Geometry check sheet. Reference: the model listing, model coordinates, mm. A direction names the side the tool comes from. Round coordinates to 2 decimals unless told otherwise and drop trailing zeros. Write each loop counter-clockwise with the first axis right and the second up, starting at its lowest first coordinate (ties: lowest second). Pieces come first, ordered by that corner, then holes.
Item 1: Cross-section at D-D (y = 2.75). Enter the section's corners in (x, z).
Item 2: Draft check along X on faces 4 (the face through (0, 17, -6)), 5 (the face through (10, 8, 4)), 6 (the face through (5.69, 7.17, 6.04)). Enter one of: pulls with the +X half, pulls with the -X half, needs draft (parallel to the pull), parting line crosses it, or undercut.
Item 3: Scan lines: probe 1 along Z at (x, y) = (8.75, 6); probe 2 along Y at (x, z) = (5, 5.7); probe 3 along Z at (x, y) = (4.85, 1.15). Record each from-to range of solid material in increasing order.
Item 4: Depth check by flat-ended pin: P1, Ø1, axis at x = -4.85, z = -1, coming from the -Y side. Enter the tip coordinate at first touch or a pass-through.
Item 5: Access from +Z, -Z, +X, -X, +Y, -Y to the whole of each face (thin tool, end or side, straight path). Record for faces 1 (the face through (4, 1, -1)), 2 (the face through (-5, 7, 6)), 3 (the face through (0, 9, -3)).
Item 6: Cross-section at A-A (z = -1). Enter the section's corners in (x, y), then the cut area to 3 significant figures.
Item 7: Cross-section at C-C (x = 4.5). Enter the section's corners in (y, z), then the cut area to 3 significant figures.
Item 8: Cross-section at B-B (y = 8.5). Enter the section's corners in (x, z).
from build123d import *

# Parameters (mm, degrees)
ESQUISSE1_W             = 20
ESQUISSE1_H             = 6
BOSS_EXTRU_1_DEPTH      = 2
ESQUISSE1_4_W           = 20
ESQUISSE1_4_H           = 6
BOSS_EXTRU_2_DEPTH      = 17
ESQUISSE1_5_W           = 20
ESQUISSE1_5_H           = 6
BOSS_EXTRU_3_DEPTH      = 17
ENL_V_MAT_EXTRU_1_REACH = 20
ESQUISSE2_R             = 1.5
ENL_V_MAT_EXTRU_2_REACH = 19
ESQUISSE3_R             = 0.85


with BuildPart() as part:
    # Esquisse1 → Boss.-Extru.1 (new body)
    with BuildSketch(Plane(origin=(0, 0, 0), x_dir=(1, 0, 0), z_dir=(0, 1, 0))):
        Rectangle(ESQUISSE1_W, ESQUISSE1_H)
    extrude(amount=BOSS_EXTRU_1_DEPTH)

    # Esquisse1_4 → Boss.-Extru.2 (add)
    with BuildSketch(Plane(origin=(0, 0, 0), x_dir=(1, 0, 0), z_dir=(0, 1, 0))):
        with Locations((0, -6)):
            Rectangle(ESQUISSE1_4_W, ESQUISSE1_4_H)
    extrude(amount=BOSS_EXTRU_2_DEPTH)

    # Esquisse1_5 → Boss.-Extru.3 (add)
    with BuildSketch(Plane(origin=(0, 0, 0), x_dir=(1, 0, 0), z_dir=(0, 1, 0))):
        with Locations((0, 6)):
            Rectangle(ESQUISSE1_5_W, ESQUISSE1_5_H)
    extrude(amount=BOSS_EXTRU_3_DEPTH)

    # Esquisse2 → Enl_v. mat.-Extru.1 (cut, up to next)
    with BuildSketch(Plane.XY.offset(9), mode=Mode.PRIVATE) as enl_v_mat_extru_1_sk1:
        with Locations((-5, 8.5)):
            Circle(ESQUISSE2_R)
    enl_v_mat_extru_1_tool1 = extrude(enl_v_mat_extru_1_sk1.sketch, amount=-ENL_V_MAT_EXTRU_1_REACH, mode=Mode.PRIVATE) & part.part
    add(enl_v_mat_extru_1_tool1.solids().sort_by_distance((-5, 8.5, 9))[0], mode=Mode.SUBTRACT)
    # Esquisse2 → Enl_v. mat.-Extru.1 (cut, up to next)
    with BuildSketch(Plane.XY.offset(9), mode=Mode.PRIVATE) as enl_v_mat_extru_1_sk2:
        with Locations((5, 8.5)):
            Circle(ESQUISSE2_R)
    enl_v_mat_extru_1_tool2 = extrude(enl_v_mat_extru_1_sk2.sketch, amount=-ENL_V_MAT_EXTRU_1_REACH, mode=Mode.PRIVATE) & part.part
    add(enl_v_mat_extru_1_tool2.solids().sort_by_distance((5, 8.5, 9))[0], mode=Mode.SUBTRACT)

    # Esquisse3 → Enl_v. mat.-Extru.2 (cut, up to next)
    with BuildSketch(Plane.XZ, mode=Mode.PRIVATE) as enl_v_mat_extru_2_sk1:
        with Locations((-4.85, -1)):
            Circle(ESQUISSE3_R)
    enl_v_mat_extru_2_tool1 = extrude(enl_v_mat_extru_2_sk1.sketch, amount=-ENL_V_MAT_EXTRU_2_REACH, mode=Mode.PRIVATE) & part.part
    add(enl_v_mat_extru_2_tool1.solids().sort_by_distance((-4.85, 0, -1))[0], mode=Mode.SUBTRACT)
    # Esquisse3 → Enl_v. mat.-Extru.2 (cut, up to next)
    with BuildSketch(Plane.XZ, mode=Mode.PRIVATE) as enl_v_mat_extru_2_sk2:
        with Locations((4.85, -1)):
            Circle(ESQUISSE3_R)
    enl_v_mat_extru_2_tool2 = extrude(enl_v_mat_extru_2_sk2.sketch, amount=-ENL_V_MAT_EXTRU_2_REACH, mode=Mode.PRIVATE) & part.part
    add(enl_v_mat_extru_2_tool2.solids().sort_by_distance((4.85, 0, -1))[0], mode=Mode.SUBTRACT)


solid = part.part
Resolved:
1. outline: (-10, -9) - (10, -9) - (10, -3) - (-10, -3) - close; (-10, 3) - (10, 3) - (10, 9) - (-10, 9) - close
2. face 4: needs draft
2. face 5: pulls with the +X half
2. face 6: undercut
3. probe 1: z = -9 to -3, 3 to 9
3. probe 2: y = 0 to 7, 10 to 17
3. probe 3: z = -9 to -1.85, -0.15 to 9
4. P1: passes through
5. face 1: +Y, -Y
5. face 2: +Z
5. face 3: +X, -X, +Y
6. outline: (-10, 0) - (-5.7, 0) - (-5.7, 2) - (-10, 2) - close; (-4, 0) - (4, 0) - (4, 2) - (-4, 2) - close; (5.7, 0) - (10, 0) - (10, 2) - (5.7, 2) - close
6. area: 33.2 mm2
7. outline: (0, -9) - (17, -9) - (17, -3) - (2, -3) - (2, -1.77) - (0, -1.77) - close; (0, -0.23) - (2, -0.23) - (2, 3) - (7.09, 3) - (7.09, 9) - (0, 9) - close; (9.91, 3) - (17, 3) - (17, 9) - (9.91, 9) - close
7. area: 196 mm2
8. outline: (-10, -9) - (10, -9) - (10, -3) - (-10, -3) - close; (-10, 3) - (-6.5, 3) - (-6.5, 9) - (-10, 9) - close; (-3.5, 3) - (3.5, 3) - (3.5, 9) - (-3.5, 9) - close; (6.5, 3) - (10, 3) - (10, 9) - (6.5, 9) - close
